from build123d import *

# Parameters (mm, degrees)
SCHIZZO1_R                    = 17.5
ESTRUSIONE_ESTRUSIONE1_DEPTH  = 50
TAGLIO_ESTRUSIONE1_REACH      = 144.171
SCHIZZO10_R                   = 16.3
TAGLIO_ESTRUSIONE3_DEPTH      = 143.170672106
TAGLIO_ESTRUSIONE3_DEPTH_BACK = 143.170672106
SCHIZZO14_R                   = 2.5
SKETCH1_R                     = 16.3
SKETCH1_R_2                   = 14.8
BOSS_EXTRUDE3_DEPTH           = 15
BOSS_EXTRUDE4_DEPTH           = 5


with BuildPart() as part:
    # Schizzo1 → Estrusione-Estrusione1 (new body)
    with BuildSketch(Plane(origin=(0, 0, 0), x_dir=(1, 0, 0), z_dir=(0, 1, 0))):
        with Locations(Location((0, 0, 0), (0, 0, 270))):
            Circle(SCHIZZO1_R)
    extrude(amount=ESTRUSIONE_ESTRUSIONE1_DEPTH)

    # Schizzo7 → Rivoluzione1 (revolve)
    with BuildSketch(Plane.XY):
        with BuildLine():
            Line((0, 140), (-2.55, 140))
            add(Edge.make_bspline(
                [(-2.55, 140), (-17.5, 113.62789219), (-17.5, 50)],
                knots=[0, 0, 0, 1, 1, 1], degree=2))
            Line((-17.5, 50), (-16.3, 50))
            add(Edge.make_bspline(
                [(-2, 138.8), (-16.3, 113.62789219), (-16.3, 50)],
                knots=[0, 0, 0, 1, 1, 1], degree=2))
            Line((-2, 138.8), (0, 138.8))
            Line((0, 138.8), (0, 140))
        make_face()
    revolve(axis=Axis((0, 50, 0), (0, 1, 0)))

    # Schizzo10 → Taglio-Estrusione1 (cut, up to next)
    with BuildSketch(Plane(origin=(0, 0, 0), x_dir=(1, 0, 0), z_dir=(0, 1, 0)), mode=Mode.PRIVATE) as taglio_estrusione1_sk1:
        with Locations(Location((0, 0, 0), (0, 0, 90))):
            Circle(SCHIZZO10_R)
    taglio_estrusione1_tool1 = extrude(taglio_estrusione1_sk1.sketch, amount=TAGLIO_ESTRUSIONE1_REACH, mode=Mode.PRIVATE) & part.part
    add(taglio_estrusione1_tool1.solids().sort_by_distance((0, 0, 0))[0], mode=Mode.SUBTRACT)

    # Schizzo14 → Taglio-Estrusione3 (cut, two sides: drawn at the far end of the back side and taken through both)
    with BuildSketch(Plane(origin=(0, 140, 0), x_dir=(1, 0, 0), z_dir=(0, 1, 0)).offset(-TAGLIO_ESTRUSIONE3_DEPTH_BACK)):
        with Locations(Location((0, 0, 0), (0, 0, 90))):
            Circle(SCHIZZO14_R)
    extrude(amount=TAGLIO_ESTRUSIONE3_DEPTH + TAGLIO_ESTRUSIONE3_DEPTH_BACK, mode=Mode.SUBTRACT)

    # Sketch1 → Boss-Extrude3 (add)
    with BuildSketch(Plane.XZ):
        with Locations(Location((0, 0, 0), (0, 0, 270))):
            Circle(SKETCH1_R)
        with Locations(Location((0, 0, 0), (0, 0, 270))):
            Circle(SKETCH1_R_2, mode=Mode.SUBTRACT)
    extrude(amount=-BOSS_EXTRUDE3_DEPTH)

    # Sketch2 → Boss-Extrude4 (add)
    with BuildSketch(Plane.XZ):
        with BuildLine():
            ThreePointArc((-14.8, 0), (-14.688451314, -1.813669762), (-14.355486756, -3.6))
            Line((-14.355486756, -3.6), (-10.845070423, -3.6))
            ThreePointArc((-10.845070423, -3.6), (-8.29948601, -2.545584412), (-7.245070423, 0))
            Line((-7.245070423, 0), (-8.645070423, 0))
            ThreePointArc((-8.645070423, 0), (-10.845070423, -2.2), (-13.045070423, 0))
            Line((-13.045070423, 0), (-14.8, 0))
        make_face()
        with BuildLine():
            Line((-10.845070423, 3.6), (-14.355486756, 3.6))
            ThreePointArc((-14.355486756, 3.6), (-14.688451314, 1.813669762), (-14.8, 0))
            Line((-14.8, 0), (-13.045070423, 0))
            ThreePointArc((-13.045070423, 0), (-10.845070423, 2.2), (-8.645070423, 0))
            Line((-8.645070423, 0), (-7.245070423, 0))
            ThreePointArc((-7.245070423, 0), (-8.29948601, 2.545584412), (-10.845070423, 3.6))
        make_face()
        with BuildLine():
            ThreePointArc((8.645070423, 0), (10.845070423, 2.2), (13.045070423, 0))
            Line((13.045070423, 0), (14.8, 0))
            ThreePointArc((14.8, 0), (14.688451314, 1.813669762), (14.355486756, 3.6))
            Line((14.355486756, 3.6), (10.845070423, 3.6))
            ThreePointArc((10.845070423, 3.6), (8.29948601, 2.545584412), (7.245070423, 0))
            Line((7.245070423, 0), (8.645070423, 0))
        make_face()
        with BuildLine():
            Line((14.8, 0), (13.045070423, 0))
            ThreePointArc((13.045070423, 0), (10.845070423, -2.2), (8.645070423, 0))
            Line((8.645070423, 0), (7.245070423, 0))
            ThreePointArc((7.245070423, 0), (8.29948601, -2.545584412), (10.845070423, -3.6))
            Line((10.845070423, -3.6), (14.355486756, -3.6))
            ThreePointArc((14.355486756, -3.6), (14.688451314, -1.813669762), (14.8, 0))
        make_face()
    extrude(amount=-BOSS_EXTRUDE4_DEPTH)


solid = part.part
Can you work these out from the model? Positions are in its coordinate system, mm. A direction names the side the tool comes from. Round coordinates to 2 decimals unless told otherwise and drop trailing zeros. Loops run counter-clockwise (first coordinate to the right, second up) from the corner with the lowest first, then second, coordinate; pieces in that order, holes last. Notation, with made-up numbers: (21, 55.5) - (77, 55.5) arc R29 ccw to (77, 82.5) - close; hole circle Ø11 at (17.25, 59). An arc over 180 degrees is marked (long way). Use CSV: the item, a comma, the result in double quotes. Start each with the question number.
1) Please list where these lines run through material, in increasing order: probe 1 along X at (y, z) = (40.5, 0.5); probe 2 along Z at (x, y) = (3, 82); probe 3 along X at (y, z) = (33.5, -4.5). Write a range as [from, to].
2) We'd pull the mould along Z, two halves only. Please class faces 4 (the flat face through (9.2, 0, -2.5)), 5 (the flat face through (-13.2, 15, -7.2)), 6 (the cylindrical face through (-10.648, 24.65, -13.887)): released by +Z, released by -Z, zero draft, split by the parting line, or undercut.
3) For pin 1 Ø1.5 at (x, z) = (4.5, 0) entering from +Y; pin 2 Ø1 at (x, y) = (-12, 73) entering from +Z; pin 3 Ø4 at (y, z) = (69.5, -8.5) entering from +X, each with a flat end and sliding along its axis, tell me the tip position at first contact or that it passes through.
4) If we section it at A-A on y = 41.5: Write out the boundary of the cut face in (x, z).
5) For faces 1 (the cylindrical face through (2.44, 138.94, 0.54)), 2 (the cylindrical face through (8.647, 2.465, -0.097)), 3 (the cylindrical face through (-5.67, 7.4, -13.67)), which set-ups out of +Z, -Z, +X, -X, +Y, -Y let a thin tool reach every point of the face, with its end or its side?
Geometry results:
1,probe 1,"x = [-17.49, -16.29], [16.29, 17.49]"
1,probe 2,"z = [-16.11, -14.93], [14.93, 16.11]"
1,probe 3,"x = [-16.91, -15.67], [15.67, 16.91]"
2,face 4,"zero draft"
2,face 5,"undercut"
2,face 6,"split by the parting line"
3,pin 1,"stops at y = 137.78"
3,pin 2,"stops at z = 12.46"
3,pin 3,"stops at x = 15.84"
4,outline,"circle Ø35 at (0, 0); hole circle Ø32.6 at (0, 0)"
5,face 1,"+Y, -Y"
5,face 2,"-Y"
5,face 3,"none"
